from build123d import *

# Parameters (mm, degrees)
F0_W          = 60
F0_H          = 70
F1_DEPTH      = 20
F3_DEPTH      = 10
F3_DEPTH_BACK = 10
F4_D          = 30
F4_DEPTH      = 35.001
F5_D          = 30
F7_D          = 8
F9_D          = 8
F11_D         = 8
F13_D         = 8


with BuildPart() as f1:
    # F0 (on Top) → F1 (new body)
    with BuildSketch(Plane.XY):
        Rectangle(F0_W, F0_H)
    extrude(amount=F1_DEPTH)

    # F2 (on Front) → F3 (join, two sides)
    with BuildSketch(Plane.XZ) as f3_sk:
        with BuildLine():
            Line((-30, 70), (-30, 20))
            Line((-30, 20), (30, 20))
            Line((30, 20), (30, 70))
            ThreePointArc((30, 70), (0, 100), (-30, 70))
        make_face()
    extrude(amount=F3_DEPTH)
    extrude(f3_sk.sketch, amount=-F3_DEPTH_BACK)

    # F4 (through all, one way)
    with BuildSketch(Plane.XZ):
        with Locations((0, 70)):
            Circle(F4_D / 2)
    extrude(amount=-F4_DEPTH, mode=Mode.SUBTRACT)

    # F5 (through all)
    with Locations(Plane(origin=(0, 0, 0), x_dir=(1, 0, 0), z_dir=(0, 1, 0))):
        with Locations((0, -70)):
            Hole(F5_D / 2)

    # F7 (through all)
    with Locations(Plane(origin=(0, 0, 0), x_dir=(1, 0, 0), z_dir=(0, 0, -1))):
        with Locations((-15.0762257692, 22.7768636146)):
            Hole(F7_D / 2)

    # F9 (through all)
    with Locations(Plane(origin=(0, 0, 0), x_dir=(1, 0, 0), z_dir=(0, 0, -1))):
        with Locations((13.9395821379, 22.5753379162)):
            Hole(F9_D / 2)

    # F11 (through all)
    with Locations(Plane(origin=(0, 0, 0), x_dir=(1, 0, 0), z_dir=(0, 0, -1))):
        with Locations((14.5101989083, -22.7402444433)):
            Hole(F11_D / 2)

    # F13 (through all)
    with Locations(Plane(origin=(0, 0, 0), x_dir=(1, 0, 0), z_dir=(0, 0, -1))):
        with Locations((-15.1346469246, -22.9134526099)):
            Hole(F13_D / 2)


solid = f1.part
Can you work these out from the model? Positions are in its coordinate system, mm. A direction names the side the tool comes from. Coordinates: 2 decimals unless noted, no trailing zeros. Loops run counter-clockwise (first coordinate to the right, second up) from the corner with the lowest first, then second, coordinate; pieces in that order, holes last. Notation, with made-up numbers: (45.5, 17) - (83.5, 17) arc R16 cw to (83.5, 41) - close; hole circle Ø10 at (-36, 62). An arc over 180 degrees is marked (long way). Answer as a JSON object with one key per item and string values. Group by question number.
Item 1: On a 3-axis mill with a long thin cutter (end or side, diameter ignored), from which of +Z, -Z, +X, -X, +Y, -Y can I reach the whole of each face in a straight line? I mean faces 1 (the face through (0, -10, 52)), 2 (the face through (0, 10, 52)), 3 (the face through (0, 35, 10)). Say none if no direction works.
Item 2: If we section it at D-D (x = 26.5): List the corners of the cut face in (y, z) for me, plus the area to 3 significant figures.
Item 3: For pin 1 (13 mm diameter, centred on x = 14.51, y = 22.74, fed in from +Z); pin 2 (1 mm diameter, centred on x = -13, z = 63.5, fed in from -Y); pin 3 (5 mm diameter, centred on x = -22.5, z = 43.5, fed in from +Y); pin 4 (1.5 mm diameter, centred on y = 11, z = 72, fed in from +X), each with a flat end and sliding along its axis, tell me the tip position at first contact or that it passes through.
Item 4: If I drill on L1, parallel to X at y = -6.25, z = 70; L2, parallel to Z at x = -21.5, y = -29; L3, parallel to Y at x = -25, z = 22.5, over which ranges is the centre line in solid material (lowest first)? Write a range as from..to.
Item 5: If we mould it in two halves opening along X, with no side actions, what happens to faces 4 (the face through (30, 0, 27)), 5 (the face through (0, -35, 10)), 6 (the face through (-11.96, 25.35, 10.14))? For each: released by +X, released by -X, zero draft, split by the parting line, or undercut.
Item 6: If we section it at A-A (x = 0): List the corners of the cut face in (y, z) for me.
Item 7: If we section it at B-B (z = 83.5): List the corners of the cut face in (x, y) for me, plus the area to 3 significant figures.
Item 8: If we section it at C-C (z = 12): List the corners of the cut face in (x, y) for me, plus the area to 3 significant figures.
Returned:
{
 "1": {"face 1": "+Z, +X, -X, -Y", "face 2": "+Z, +X, -X, +Y", "face 3": "+Z, -Z, +X, -X, +Y"},
 "2": {"outline": "(-35, 0) - (35, 0) - (35, 20) - (10, 20) - (10, 84.06) - (-10, 84.06) - (-10, 20) - (-35, 20) - close", "area": "2,680 mm²"},
 "3": {"pin 1": "stops at z = 20", "pin 2": "stops at y = -10", "pin 3": "stops at y = 10", "pin 4": "passes through"},
 "4": {"L1": "x = -30..-15, 15..30", "L2": "z = 0..20", "L3": "y = -10..10"},
 "5": {"face 4": "released by +X", "face 5": "zero draft", "face 6": "undercut"},
 "6": {"outline": "(-35, 0) - (35, 0) - (35, 20) - (10, 20) - (10, 55) - (-10, 55) - (-10, 20) - (-35, 20) - close; (-10, 85) - (10, 85) - (10, 100) - (-10, 100) - close"},
 "7": {"outline": "(-26.79, -10) - (-6.54, -10) - (-6.54, 10) - (-26.79, 10) - close; (6.54, -10) - (26.79, -10) - (26.79, 10) - (6.54, 10) - close", "area": "810 mm²"},
 "8": {"outline": "(-30, -35) - (30, -35) - (30, 35) - (-30, 35) - close; hole circle Ø8 at (-15.13, 22.91); hole circle Ø8 at (-15.08, -22.78); hole circle Ø8 at (13.94, -22.58); hole circle Ø8 at (14.51, 22.74)", "area": "4,000 mm²"}
}
